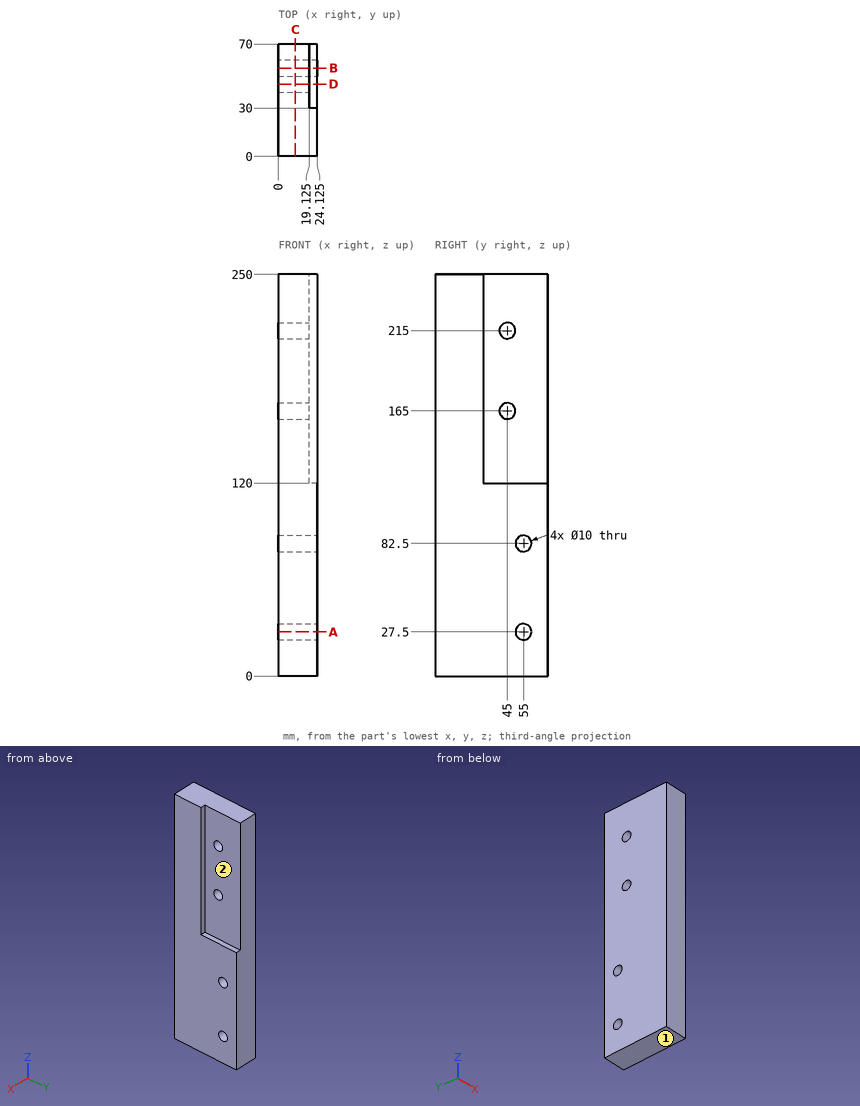
Job drawing, mm, ordinate dimensions from the low corner. One solid piece. A direction names the side the tool comes from. Coordinates: 2 decimals unless noted, no trailing zeros. Order: outer loops, then holes, each group sorted by start corner. A loop starts at its lowest first (then second) coordinate and runs counter-clockwise, first axis right, second up. Notation, with made-up numbers: (2.5, 72.5) -> (55.5, 72.5) arc R26 cw to (55.5, 87.5) -> close; hole circle Ø3 at (17.25, -2). An arc over 180 degrees is marked (long way). Return JSON: item names as keys, results as strings. Group by question number.
Item 1: Saw through at D-D on y = 45. Write the cut outline in (x, z) (3 decimals), then the cut area to 3 significant figures.
Item 2: Flat gauge pins, fed straight in: P1, Ø8, axis at y = 45, z = 165, coming from the -X side; P2, Ø11.5, axis at y = 45, z = 215, coming from the +X side (3 decimals). Where does each tip first touch, or does it go through?
Item 3: Saw through at C-C on x = 10.5. Write the cut outline in (y, z).
Item 4: Wall check: line 1 along Z through (x, y) = (22.5, 55.5); line 2 along Z through (x, y) = (12, 45); line 3 along X through (y, z) = (31, 170) (3 decimals). Give the ranges that are in metal, low to high. Write a range as [from, to].
Item 5: Tool access for the marked faces 1 and 2: list every direction of +Z, -Z, +X, -X, +Y, -Y with a clear straight run to the whole face (end or side of a thin tool).
Item 6: Saw through at B-B on y = 55. Write the cut outline in (x, z) (3 decimals).
Item 7: Saw through at A-A on z = 27.5. Write the cut outline in (x, y) (3 decimals).
Values found:
{
 "1": {"outline": "(0, 0) -> (24.125, 0) -> (24.125, 120) -> (19.125, 120) -> (19.125, 160) -> (0, 160) -> close; (0, 170) -> (19.125, 170) -> (19.125, 210) -> (0, 210) -> close; (0, 220) -> (19.125, 220) -> (19.125, 250) -> (0, 250) -> close", "area": "5,000 mm2"},
 "2": {"P1": "passes through", "P2": "stops at x = 19.125"},
 "3": {"outline": "(0, 0) -> (70, 0) -> (70, 250) -> (0, 250) -> close; hole circle Ø10 at (45, 165); hole circle Ø10 at (45, 215); hole circle Ø10 at (55, 27.5); hole circle Ø10 at (55, 82.5)"},
 "4": {"line 1": "z = [0, 22.53], [32.47, 77.53], [87.47, 120]", "line 2": "z = [0, 160], [170, 210], [220, 250]", "line 3": "x = [0, 19.125]"},
 "5": {"face 1": "-Z, +X, -X, +Y, -Y", "face 2": "+Z, +X, +Y"},
 "6": {"outline": "(0, 0) -> (24.125, 0) -> (24.125, 22.5) -> (0, 22.5) -> close; (0, 32.5) -> (24.125, 32.5) -> (24.125, 77.5) -> (0, 77.5) -> close; (0, 87.5) -> (24.125, 87.5) -> (24.125, 120) -> (19.125, 120) -> (19.125, 250) -> (0, 250) -> close"},
 "7": {"outline": "(0, 0) -> (24.125, 0) -> (24.125, 50) -> (0, 50) -> close; (0, 60) -> (24.125, 60) -> (24.125, 70) -> (0, 70) -> close"}
}
